Verification items for this drawing (mm, ordinates from the low corner). Round coordinates to 2 decimals unless told otherwise and drop trailing zeros. Loops run counter-clockwise (first coordinate to the right, second up) from the corner with the lowest first, then second, coordinate; pieces in that order, holes last. Notation, with made-up numbers: (78, 55) -> (107, 55) arc R14 ccw to (107, 60) -> close; hole circle Ø7 at (47.25, -8). An arc over 180 degrees is marked (long way). Use a Markdown table: item, result. Add a question column.
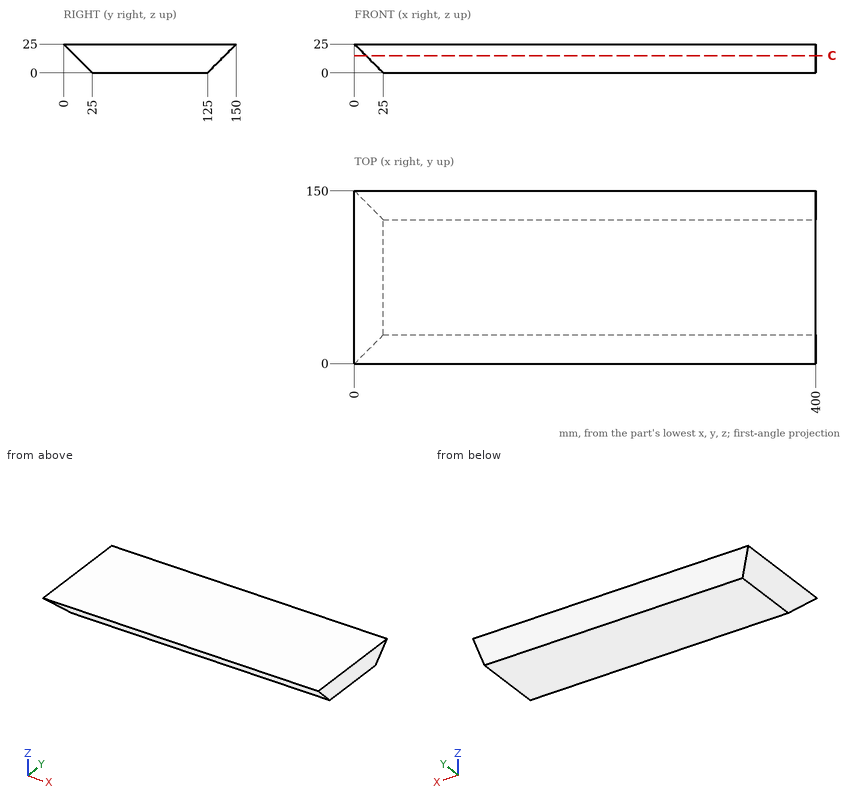
1) Thickness scan on line 1 (Z direction, x = 275.5, y = 132); line 2 (Y direction, x = 201, z = 18.25); line 3 (Y direction, x = 202.5, z = 14). Record the ranges inside material, lowest first.
2) Go/stop test with flat-tipped pins: pin 1 (6 mm diameter, centred on x = 292.5, z = 9, fed in from -Y); pin 2 (12 mm diameter, centred on x = 218, z = 17.5, fed in from +Y); pin 3 (4 mm diameter, centred on x = 357.5, z = 17, fed in from -Y). Record where each tip stops, or that it passes through.
3) Sectioned sample at C-C on z = 15. Enter the section's corners in (x, y).
Geometry results:
| question | item | result |
|---|---|---|
| 1 | line 1 | 7 to 25 |
| 1 | line 2 | 6.75 to 143.25 |
| 1 | line 3 | 11 to 139 |
| 2 | pin 1 | y = 13 |
| 2 | pin 2 | y = 148.5 |
| 2 | pin 3 | y = 6 |
| 3 | outline | (10, 10) -> (400, 10) -> (400, 140) -> (10, 140) -> close |
